Read the model definition and answer for the solid it produces. Units are mm, in the model's axes. Face numbers are marked on the shaded views. A direction names the side the tool comes from. Coordinates: 2 decimals unless noted, no trailing zeros. Write each loop counter-clockwise with the first axis right and the second up, starting at its lowest first coordinate (ties: lowest second). Pieces come first, ordered by that corner, then holes. Notation, with made-up numbers: M -36.5,-31.5 L -29.5,-31.5 A21 ccw -29.5,-8.5 Z; hole C -23.75,54.5 d11. An arc over 180 degrees is marked long. Write item = value, one per line.
from build123d import *

# Parameters (mm, degrees)
SKETCH_1_R                  = 6.5
EXTRUDE_1_DEPTH             = 26
SKETCH_2_R                  = 2.85
CUT_EXTRUDE_1_DEPTH         = 3.5
HOLE_WIZARD_M32_D           = 3.4
HOLE_WIZARD_M32_CSINK_D     = 6.3
HOLE_WIZARD_M32_CSINK_ANGLE = 90


with BuildPart() as part:
    # Эскиз1 → Бобышка-Вытянуть1 (new body)
    with BuildSketch(Plane(origin=(0, 0, 0), x_dir=(1, 0, 0), z_dir=(0, 1, 0))):
        with Locations(Location((0, 0, 0), (0, 0, 90))):
            Circle(SKETCH_1_R)
    extrude(amount=EXTRUDE_1_DEPTH)

    # Эскиз2 → Вырез-Вытянуть1 (cut)
    with BuildSketch(Plane.XZ):
        with Locations(Location((0, 0, 0), (0, 0, 270))):
            Circle(SKETCH_2_R)
    extrude(amount=-CUT_EXTRUDE_1_DEPTH, mode=Mode.SUBTRACT)

    # Зенковка для  винта с плоской головкой M32 (through all)
    with Locations(Plane(origin=(0, 26, 0), x_dir=(1, 0, 0), z_dir=(0, 1, 0))):
        with Locations((0, 0)):
            CounterSinkHole(HOLE_WIZARD_M32_D / 2, HOLE_WIZARD_M32_CSINK_D / 2, counter_sink_angle=HOLE_WIZARD_M32_CSINK_ANGLE)

    # Вырез-По траектории2: sweep along a path in Эскиз5
    with BuildLine(Plane(origin=(0, 18, 0), x_dir=(-1, 0, 0), z_dir=(0, -1, 0))) as sweep_2_path:
        CenterArc((0, 0), 6.5, 0, 360)
    # Эскиз6 → Вырез-По траектории2 (sweep, cut)
    with BuildSketch(Plane(origin=(0, 0, 0), x_dir=(0, 0, -1), z_dir=(1, 0, 0))):
        Polygon((6.5, 19), (5.5, 18), (6.5, 17), align=None)
    sweep(path=sweep_2_path.line, mode=Mode.SUBTRACT)


solid = part.part
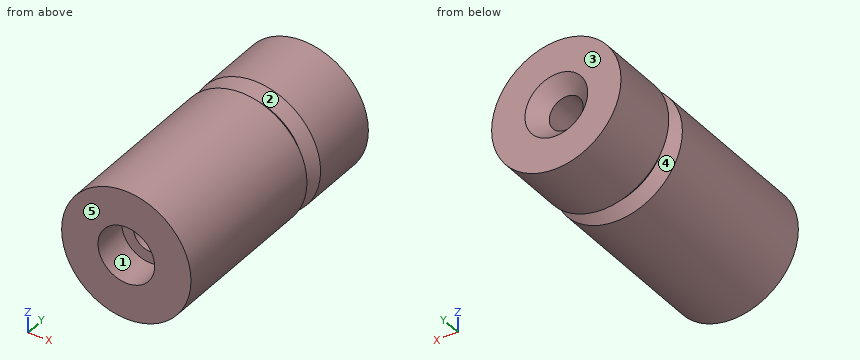
Item 1: Flat-ended cylindrical pins translate along their axes: pin 1 (1.5 mm diameter, centred on y = 20, z = -2, fed in from -X); pin 2 (5.5 mm diameter, centred on x = 0, z = 0, fed in from -Y); pin 3 (2 mm diameter, centred on x = -4, y = 16, fed in from +Z). Find the tip coordinate at first contact, or state that the pin passes through.
Worked answers:
pin_1 = -6.38
pin_2 = 3.5
pin_3 = 5.77
Item 2: Consider line 1 along X through (y, z) = (1.8, 0); line 2 along Y through (x, z) = (-5.5, -1.5); line 3 along Z through (x, y) = (0.75, 20). Determine where each line is inside the solid, lowest interval first. Write a range as from..to.
Worked answers:
line_1 = -6.5..-2.85, 2.85..6.5
line_2 = 0..17.8, 18.2..26
line_3 = -6.46..-1.53, 1.53..6.46
Item 3: Find section B-B (z = 0). Determine the outline of the cut face in (x, y), and give its area (3 significant figures).
Worked answers:
outline = M -6.5,0 L -2.85,0 L -2.85,3.5 L -1.7,3.5 L -1.7,24.55 L -3.15,26 L -6.5,26 L -6.5,19 L -5.5,18 L -6.5,17 Z; M 1.7,3.5 L 2.85,3.5 L 2.85,0 L 6.5,0 L 6.5,17 L 5.5,18 L 6.5,19 L 6.5,26 L 3.15,26 L 1.7,24.55 Z
area = 237 mm²
Item 4: For a pull along Y with two mould halves and no side action, classify the marked faces 1, 2 and 3 as released by +Y, released by -Y, zero draft, split by the parting line, or undercut.
Worked answers:
face_1 = zero draft
face_2 = undercut
face_3 = released by +Y
Item 5: Which of the six approach directions +Z, -Z, +X, -X, +Y, -Y give full straight-line access (tool end or side, diameter ignored) to the marked faces 4 and 5?
Worked answers:
face_4 = none
face_5 = +Z, -Z, +X, -X, -Y
Item 6: Find section A-A (x = 0). Determine the outline of the cut face in (y, z), and give its area (3 significant figures).
Worked answers:
outline = M 0,-6.5 L 17,-6.5 L 18,-5.5 L 19,-6.5 L 26,-6.5 L 26,-3.15 L 24.55,-1.7 L 3.5,-1.7 L 3.5,-2.85 L 0,-2.85 Z; M 0,2.85 L 3.5,2.85 L 3.5,1.7 L 24.55,1.7 L 26,3.15 L 26,6.5 L 19,6.5 L 18,5.5 L 17,6.5 L 0,6.5 Z
area = 237 mm²
